Read the model definition and answer for the solid it produces. Units are mm, in the model's axes. Face numbers are marked on the shaded views. A direction names the side the tool comes from. Give positions to 0.01 mm unless a question says otherwise; leave off trailing zeros. Write each loop counter-clockwise with the first axis right and the second up, starting at its lowest first coordinate (ties: lowest second). Pieces come first, ordered by that corner, then holes. Notation, with made-up numbers: M -16.5,88 L 42.5,88 A16 ccw 42.5,118 Z; hole C 26,86.25 d11. An arc over 180 degrees is marked long. Use a Markdown table: item, result. Add a question column.
Item 1: For the marked faces 1 and 2, determine the directions among +Z, -Z, +X, -X, +Y, -Y from which every point of the face is accessible in a straight line to the end or side of a thin tool.
Item 2: A cutting plane is placed at C-C on z = -5.25. Determine the outline of the cut face in (x, y), then the cut area to 3 significant figures.
Item 3: Given P1, Ø3, axis at x = -2.5, z = -8.5, coming from the +Y side; P2, Ø1, axis at x = 0, z = -10.5, coming from the +Y side, each flat-ended and moving along its own axis, determine where each tip first touches the part or whether it passes through.
Item 4: Consider probe 1 along Z at (x, y) = (-0.75, -2.75); probe 2 along Y at (x, z) = (0, -6.25); probe 3 along X at (y, z) = (1, -11). Determine where each line is inside the solid, lowest interval first. Write a range as [from, to].
Autodesk Inventor part; units mm, degrees
ref_plane "YZ Plane" through (0, 0, 0) normal (1, 0, 0) x (0, 1, 0)
ref_plane "XZ Plane" through (0, 0, 0) normal (0, 1, 0) x (-1, 0, 0)
ref_plane "XY Plane" through (0, 0, 0) normal (0, 0, 1) x (1, 0, 0)
sketch "スケッチ1" plane through (0, 0, 0) normal (0, 0, 1) x (1, 0, 0)
  circle A0 centre (0, 0) radius 3.5
  dimension "d0" = 7
extrude "押し出し1" add sketch "スケッチ1" along normal blind 0.7
sketch "スケッチ2" plane through (0, 0, 0) normal (0, 0, -1) x (-1, 0, 0)
  circle A0 centre (0, 0) radius 1.5
  dimension "d3" = 3
extrude "押し出し2" add sketch "スケッチ2" along normal blind 12
thread "ねじ1"
fillet "フィレット1" radius 0.7 1 edges at (-3.5, 0, 0.7)
properties part number "ネジ低頭m3.12" material "鋼、高強度、低合金"
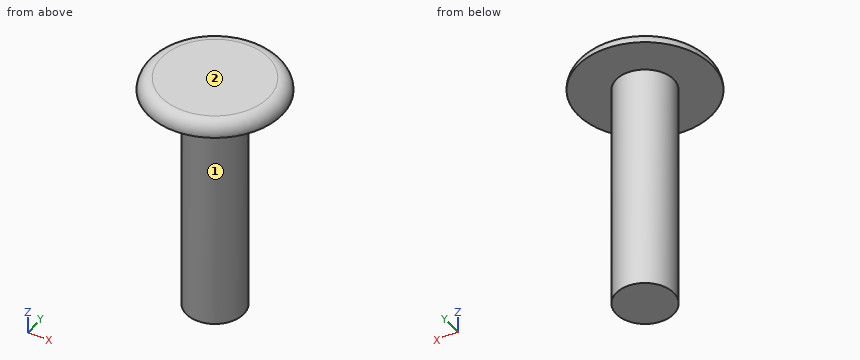
Filled in:
| question | item | result |
|---|---|---|
| 1 | face 1 | -Z |
| 1 | face 2 | +Z, +X, -X, +Y, -Y |
| 2 | outline | C 0,0 d3 |
| 2 | area | 7.07 mm² |
| 3 | P1 | y = 1.12 |
| 3 | P2 | y = 1.5 |
| 4 | probe 1 | [0, 0.7] |
| 4 | probe 2 | [-1.5, 1.5] |
| 4 | probe 3 | [-1.12, 1.12] |
